Part model, mm, in its own coordinate system. A direction names the side the tool comes from. Round coordinates to 2 decimals unless told otherwise and drop trailing zeros. Write each loop counter-clockwise with the first axis right and the second up, starting at its lowest first coordinate (ties: lowest second). Pieces come first, ordered by that corner, then holes.
```python
from build123d import *

# Parameters (mm, degrees)
SKETCH002_R     = 2
PAD_DEPTH       = 4
PAD001_DEPTH    = 5
SKETCH004_R     = 0.75
POCKET001_DEPTH = 5


with BuildPart() as part:
    # Sketch002 → Pad (new body)
    with BuildSketch(Plane.XZ):
        Circle(SKETCH002_R)
    extrude(amount=PAD_DEPTH)

    # Sketch003 (on Face2 of Pad) → Pad001 (join)
    with BuildSketch(Plane(origin=(0, 0, 0), x_dir=(1, 0, 0), z_dir=(0, 1, 0))):
        with BuildLine():
            Line((-1.85405, 0.75), (1.85405, 0.75))
            ThreePointArc((1.85405, -0.75), (2, 0), (1.85405, 0.75))
            Line((1.85405, -0.75), (-1.85405, -0.75))
            ThreePointArc((-1.85405, 0.75), (-2, 0), (-1.85405, -0.75))
        make_face()
    extrude(amount=PAD001_DEPTH)

    # Sketch004 (on Face2 of Pad001) → Pocket001 (cut)
    with BuildSketch(Plane(origin=(0, 0, -0.75), x_dir=(1, 0, 0), z_dir=(0, 0, -1))):
        with Locations((0, -3.4)):
            Circle(SKETCH004_R)
    extrude(amount=-POCKET001_DEPTH, mode=Mode.SUBTRACT)


with BuildPart() as part_1:
    # Body001 placement: moved
    add(part.part.moved(Location((0, 48, 6))))


solid = part_1.part
```
Q1. Cut at C-C on x = -1.65. Write the cut outline in (y, z).
Values follow:
outline: (44, 4.87) - (48, 4.87) - (48, 5.25) - (53, 5.25) - (53, 6.75) - (48, 6.75) - (48, 7.13) - (44, 7.13) - close
Q2. Mould opens along Y. For faces 1 (the flat face through (0, 44, 6)), 2 (the flat face through (0, 53, 6)), 3 (the flat face through (0, 50, 6.75)), 4 (the cylindrical face through (0.346, 52.065, 5.99)) say: +Y half, -Y half, draft (parallel to the pull), parting line (faces both ways), or undercut.
Values follow:
face 1: -Y half
face 2: +Y half
face 3: draft
face 4: undercut
Q3. Cut at A-A on x = 0.05. Write the cut outline in (y, z), plus the area to 4 significant figures.
Values follow:
outline: (44, 4) - (48, 4) - (48, 5.25) - (50.65, 5.25) - (50.65, 6.75) - (48, 6.75) - (48, 8) - (44, 8) - close; (52.15, 5.25) - (53, 5.25) - (53, 6.75) - (52.15, 6.75) - close
area: 21.25 mm2
Q4. Cut at B-B on y = 51. Write the cut outline in (x, z).
Values follow:
outline: (-1.85, 5.25) - (-0.63, 5.25) - (-0.63, 6.75) - (-1.85, 6.75) arc R2 ccw to start; (0.63, 5.25) - (1.85, 5.25) arc R2 ccw to (1.85, 6.75) - (0.63, 6.75) - close
Q5. Which spindle directions (+Z, -Z, +X, -X, +Y, -Y) get a long thin tool onto all of the face, cutting with end or side? Do faces 5 (the flat face through (0, 48, 7)), 6 (the flat face through (0, 48, 5)). Say none if no direction does.
Values follow:
face 5: +Z, +X, -X, +Y
face 6: -Z, +X, -X, +Y
Q6. Cut at D-D on z = 4.8. Write the cut outline in (x, y), plus the area to 3 significant figures.
Values follow:
outline: (-1.6, 44) - (1.6, 44) - (1.6, 48) - (-1.6, 48) - close
area: 12.8 mm2
Q7. Drop flat-ended pins along their axis: pin 1 (0.6 mm diameter, centred on x = 0.5, z = 4.5, fed in from +Y); pin 2 (1.5 mm diameter, centred on y = 46, z = 6.5, fed in from +X); pin 3 (1.1 mm diameter, centred on x = 0.5, y = 50, fed in from +Z); pin 4 (1 mm diameter, centred on x = -1, y = 46, fed in from +Z). Give the stop position or say it passes through.
Values follow:
pin 1: stops at y = 48
pin 2: stops at x = 2
pin 3: stops at z = 6.75
pin 4: stops at z = 7.94
Q8. Wall check: L1, parallel to X at y = 51.4, z = 5.95; L2, parallel to Y at x = 0, z = 5.85; L3, parallel to Z at x = 1.65, y = 49.25. Give the ranges that are in metal, low to high.
Values follow:
L1: x = -2 to -0.75, 0.75 to 2
L2: y = 44 to 50.65, 52.15 to 53
L3: z = 5.25 to 6.75
